The model under review builds one solid part; all positions refer to its coordinate system, in mm. A direction names the side the tool comes from. Give positions to 0.01 mm unless a question says otherwise; leave off trailing zeros. Order: outer loops, then holes, each group sorted by start corner. A loop starts at its lowest first (then second) coordinate and runs counter-clockwise, first axis right, second up. Notation, with made-up numbers: M 20,-13.75 L 32,-13.75 A15 cw 32,7.25 Z; hole C 69,25 d8. An arc over 180 degrees is marked long. One line per question, with ' | ' between items. Start each with the question number.
1. Wall thickness on L1, parallel to Z at x = -59.5, y = 29; L2, parallel to Y at x = -25.5, z = -22; L3, parallel to X at y = -2, z = 3.5: over which ranges is each line inside the solid? List them lowest first.
2. We need section B-B on y = 18.5. Write out the cut boundary in (x, z), then the cut area to 3 significant figures.
3. We need section D-D on x = -49. Write out the cut boundary in (y, z).
4. Insertion check: P1, Ø1.5, axis at x = -35.5, y = 16.5, coming from the -Z side; P2, Ø19, axis at x = 21, y = 15, coming from the -Z side; P3, Ø1, axis at x = -26, z = -17, coming from the +Y side. Each pin has a flat end and moves straight along its axis. Give the tip position at first contact, or say it passes through.
5. For faces 1 (the face through (63.106, -1.427, -0.415)), 2 (the face through (-1, 20, 17)), list the 3-axis set-ups (+Z, -Z, +X, -X, +Y, -Y) from which the entire face can be reached by the end or side of a thin tool; tool diameter is ignored.
6. We need section C-C on z = 15.5. Write out the cut boundary in (x, y).
7. We need section A-A on x = -18. Write out the cut boundary in (y, z), then the cut area to 3 significant figures.
```python
from build123d import *

# Parameters (mm, degrees)
SKETCH1_W                    = 152
SKETCH1_H                    = 50
BASE_FLANGE1_DEPTH           = 8
EDGE_FLANGE1_STRIP_W         = 48
EDGE_FLANGE1_STRIP_H         = 8
EDGE_FLANGE1_STRIP_CUT_DEPTH = 152
EDGE_FLANGE1_DEPTH           = 152
CHAMFER1_SIZE                = 43
CHAMFER1_SIZE2               = 30.108924143
MIRROR3_START                = 51.931179512
MIRROR3_OUTLINE_W            = 56
MIRROR3_OUTLINE_H            = 41
MIRROR3_DEPTH                = 24.663786763


# Read off the part's stored shape, not the designer's step: Mirror3
# Sheet-metal steps are written as plain solids
with BuildPart() as part:
    # Sketch1 → Base-Flange1 (new body)
    with BuildSketch(Plane(origin=(0, 0, 0), x_dir=(1, 0, 0), z_dir=(0, 1, 0))):
        Rectangle(SKETCH1_W, SKETCH1_H)
    extrude(amount=-BASE_FLANGE1_DEPTH)

    # Edge-Flange1 strip (across the edge) → Edge-Flange1 strip cut (cut)
    with BuildSketch(Plane(origin=(-76, 0, 25), x_dir=(0, 0, -1), z_dir=(1, 0, 0))):
        with Locations((-8, -4)):
            Rectangle(EDGE_FLANGE1_STRIP_W, EDGE_FLANGE1_STRIP_H)
    extrude(amount=EDGE_FLANGE1_STRIP_CUT_DEPTH, mode=Mode.SUBTRACT)

    # Edge-Flange1 section (across the edge) → Edge-Flange1 (add)
    with BuildSketch(Plane(origin=(-76, 0, 25), x_dir=(0, 0, -1), z_dir=(1, 0, 0))):
        with BuildLine():
            Line((0, 8), (0, 32))
            Line((0, 32), (8, 32))
            Line((8, 32), (8, 8))
            ThreePointArc((8, 8), (10.343145751, 2.343145751), (16, 0))
            Line((16, 0), (16, -8))
            ThreePointArc((16, -8), (4.686291501, -3.313708499), (0, 8))
        make_face()
    extrude(amount=EDGE_FLANGE1_DEPTH)

    # Chamfer1
    chamfer1_edges = [part.edges().sort_by_distance(p)[0] for p in [
        (-76, -4, -25),
    ]]
    chamfer1_side = [part.faces().sort_by_distance(p)[0] for p in [
        (-76, -0.640312424, -8),
    ]]
    chamfer(chamfer1_edges, length=CHAMFER1_SIZE, length2=CHAMFER1_SIZE2, reference=chamfer1_side[0])

    # Mirror3 outline → Mirror3 (cut)
    with BuildSketch(Plane(origin=(0, 0, 0), x_dir=(0.5735764363510512, 0, 0.8191520442889882), z_dir=(0.8191520442889882, 0, -0.5735764363510512)).offset(MIRROR3_START)):
        with Locations((32, -12.5)):
            Rectangle(MIRROR3_OUTLINE_W, MIRROR3_OUTLINE_H)
    extrude(amount=MIRROR3_DEPTH, mode=Mode.SUBTRACT)


solid = part.part
```
Entries:
1) L1: z = 17 to 25 | L2: y = -8 to 0 | L3: x = -65.85 to 65.85
2) outline: M -76,18 L -75.3,17 L 75.3,17 L 76,18 L 76,25 L -76,25 Z | area: 1,220 mm^2
3) outline: M -8,-20.56 L 0,-20.56 L 0,9 A8 cw 8,17 L 32,17 L 32,25 L 8,25 A16 ccw -8,9 Z
4) P1: stops at z = 17 | P2: stops at z = 16.6 | P3: stops at y = 0
5) face 1: -Z, +X, +Y, -Y | face 2: -Z, +X, -X, +Y
6) outline: M -74.25,-6.62 L 74.25,-6.62 L 74.25,3.34 L -74.25,3.34 Z
7) outline: M -8,-25 L 0,-25 L 0,9 A8 cw 8,17 L 32,17 L 32,25 L 8,25 A16 ccw -8,9 Z | area: 615 mm^2
